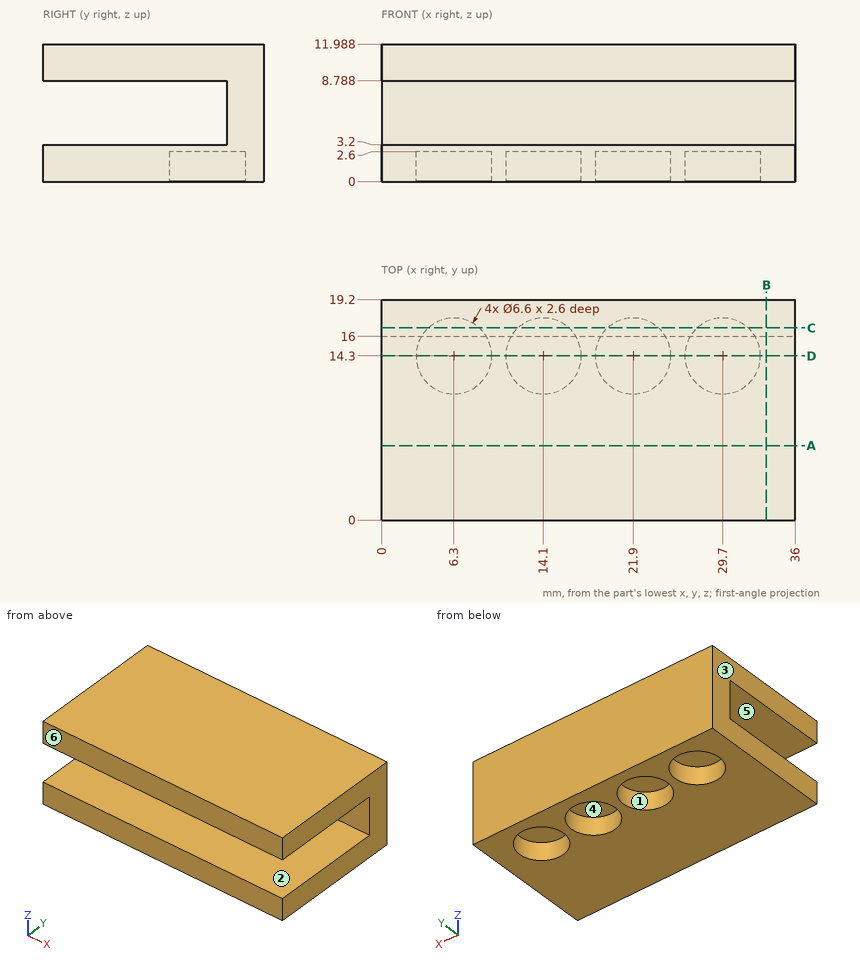
Job drawing, mm, ordinate dimensions from the low corner. One solid piece. A direction names the side the tool comes from. Round coordinates to 2 decimals unless told otherwise and drop trailing zeros. Order: outer loops, then holes, each group sorted by start corner. A loop starts at its lowest first (then second) coordinate and runs counter-clockwise, first axis right, second up. Notation, with made-up numbers: (-18.75, 73.25) -> (5.25, 73.25) arc R16 ccw to (5.25, 77.25) -> close; hole circle Ø6 at (50, 85.25). An arc over 180 degrees is marked (long way). Answer in a Markdown table with one row per item.
1) Band-saw the part on A-A on y = 6.5. Give the cut face in (x, z), and give its area (3 significant figures).
Values:
| item | result |
|---|---|
| outline | (0, 0) -> (36, 0) -> (36, 3.2) -> (0, 3.2) -> close; (0, 8.79) -> (36, 8.79) -> (36, 11.99) -> (0, 11.99) -> close |
| area | 230 mm2 |
2) Band-saw the part on D-D on y = 14.3. Give the cut face in (x, z).
Values:
| item | result |
|---|---|
| outline | (0, 0) -> (3, 0) -> (3, 2.6) -> (9.6, 2.6) -> (9.6, 0) -> (10.8, 0) -> (10.8, 2.6) -> (17.4, 2.6) -> (17.4, 0) -> (18.6, 0) -> (18.6, 2.6) -> (25.2, 2.6) -> (25.2, 0) -> (26.4, 0) -> (26.4, 2.6) -> (33, 2.6) -> (33, 0) -> (36, 0) -> (36, 3.2) -> (0, 3.2) -> close; (0, 8.79) -> (36, 8.79) -> (36, 11.99) -> (0, 11.99) -> close |
3) Wall check: L1, parallel to Z at x = 14.5, y = 10.5; L2, parallel to Y at x = 29.7, z = 1.25; L3, parallel to Z at x = 20, y = 15.5. Give the ranges that are in metal, low to high.
Values:
| item | result |
|---|---|
| L1 | 0 to 3.2, 8.79 to 11.99 |
| L2 | 0 to 11, 17.6 to 19.2 |
| L3 | 2.6 to 3.2, 8.79 to 11.99 |
4) Band-saw the part on C-C on y = 16.75. Give the cut face in (x, z), and give its area (3 significant figures).
Values:
| item | result |
|---|---|
| outline | (0, 0) -> (4.09, 0) -> (4.09, 2.6) -> (8.51, 2.6) -> (8.51, 0) -> (11.89, 0) -> (11.89, 2.6) -> (16.31, 2.6) -> (16.31, 0) -> (19.69, 0) -> (19.69, 2.6) -> (24.11, 2.6) -> (24.11, 0) -> (27.49, 0) -> (27.49, 2.6) -> (31.91, 2.6) -> (31.91, 0) -> (36, 0) -> (36, 11.99) -> (0, 11.99) -> close |
| area | 386 mm2 |
5) Pin check, flat tips, straight feed: P1, Ø1.5, axis at y = 10, z = 6.5, coming from the +X side (3 decimals); P2, Ø3.5, axis at x = 28.5, y = 15, coming from the -Z side; P3, Ø1.7, axis at x = 24.5, z = 6, coming from the -Y side. Stop position of each tip, or through.
Values:
| item | result |
|---|---|
| P1 | through |
| P2 | z = 2.6 |
| P3 | y = 16 |
6) Which spindle directions (+Z, -Z, +X, -X, +Y, -Y) get a long thin tool onto all of the face, cutting with end or side? Do the marked faces 4, 5 and 6. Say none if no direction does.
Values:
| item | result |
|---|---|
| face 4 | -Z |
| face 5 | +X, -X, -Y |
| face 6 | +Z, -Z, +X, -X, -Y |
7) Mould opens along X. For the marked faces 1, 2 and 3 say: released by +X, released by -X, zero draft, split by the parting line, or undercut.
Values:
| item | result |
|---|---|
| face 1 | undercut |
| face 2 | zero draft |
| face 3 | released by -X |
8) Band-saw the part on B-B on x = 33.5. Give the cut face in (y, z).
Values:
| item | result |
|---|---|
| outline | (0, 0) -> (19.2, 0) -> (19.2, 11.99) -> (0, 11.99) -> (0, 8.79) -> (16, 8.79) -> (16, 3.2) -> (0, 3.2) -> close |
